Check sheet for the modelled part. Datum: model origin and axes. Units: mm. A direction names the side the tool comes from. Coordinates: 2 decimals unless noted, no trailing zeros. Loops run counter-clockwise (first coordinate to the right, second up) from the corner with the lowest first, then second, coordinate; pieces in that order, holes last. Notation, with made-up numbers: M 3,-31 L 30,-31 A22 cw 30,-19 Z; hole C -40,15.5 d8. An arc over 180 degrees is marked long. Answer in a Markdown table with one row per item. Add a question column.
```python
from build123d import *

# Parameters (mm, degrees)
BOSS_EXTRUDE2_DEPTH = 65
SKETCH4_W           = 20
SKETCH4_H           = 30
CUT_EXTRUDE1_DEPTH  = 35
SKETCH5_W           = 50
SKETCH5_H           = 80
BOSS_EXTRUDE3_DEPTH = 30
SKETCH6_W           = 30
SKETCH6_H           = 25
CUT_EXTRUDE2_DEPTH  = 20
LOFT3_START         = -65
LOFT3_DEPTH         = 65
LOFT3_START_2       = 25
LOFT3_2_DEPTH       = 76


with BuildPart() as part:
    # Sketch3 → Boss-Extrude2 (new body)
    with BuildSketch(Plane.XY):
        Polygon((0, 0), (100, 0), (100, 20), (25, 20), (25, 80), (0, 80), align=None)
    extrude(amount=-BOSS_EXTRUDE2_DEPTH)

    # Sketch4 → Cut-Extrude1 (cut)
    with BuildSketch(Plane(origin=(0, 80, 0), x_dir=(1, 0, 0), z_dir=(0, 1, 0))):
        with Locations((15, 50)):
            Rectangle(SKETCH4_W, SKETCH4_H)
    extrude(amount=-CUT_EXTRUDE1_DEPTH, mode=Mode.SUBTRACT)

    # Sketch5 → Boss-Extrude3 (add)
    with BuildSketch(Plane.ZY):
        with Locations((-40, 40)):
            Rectangle(SKETCH5_W, SKETCH5_H)
    extrude(amount=BOSS_EXTRUDE3_DEPTH)

    # Sketch6 → Cut-Extrude2 (cut)
    with BuildSketch(Plane(origin=(25, 0, 0), x_dir=(0, 0, -1), z_dir=(1, 0, 0))):
        with Locations((50, 32.5)):
            Rectangle(SKETCH6_W, SKETCH6_H)
    extrude(amount=-CUT_EXTRUDE2_DEPTH, mode=Mode.SUBTRACT)

    # Loft3: read off the stored shape, not the designer's step
    # Loft3 outline → Loft3 (add)
    with BuildSketch(Plane.XY.offset(LOFT3_START)):
        Polygon((5, 45), (5, 20), (100, 20), (50, 45), align=None)
    extrude(amount=LOFT3_DEPTH)

    # Loft3 2 outline → Loft3 2 (cut)
    with BuildSketch(Plane.YZ.offset(LOFT3_START_2)):
        Polygon((20, 0), (45, -35), (45, 0), align=None)
    extrude(amount=LOFT3_2_DEPTH, mode=Mode.SUBTRACT)


solid = part.part
```
Q1. Thickness scan on L1, parallel to Y at x = 8, z = -62; L2, parallel to X at y = 45, z = -31; L3, parallel to Z at x = 18, y = 48.5. Record the ranges inside material, lowest first.
Q2. Cross-section at D-D (y = 34.5). Record the cut outline in (x, z).
Q3. Cross-section at B-B (x = 21.5). Record the cut outline in (y, z), plus the area to 3 significant figures.
Q4. Cross-section at A-A (y = 75). Record the cut outline in (x, z), plus the area to 4 significant figures.
Q5. Go/stop test with flat-tipped pins: pin 1 (1.5 mm diameter, centred on x = 26, z = -27.5, fed in from -Y); pin 2 (7.5 mm diameter, centred on y = 23.5, z = -5.5, fed in from -X); pin 3 (15 mm diameter, centred on y = 68, z = -49.5, fed in from +X); pin 4 (10.5 mm diameter, centred on y = 43, z = -11.5, fed in from +X). Record where each tip stops, or that it passes through.
Q6. Access from +Z, -Z, +X, -X, +Y, -Y to the whole of each face (thin tool, end or side, straight path). Record for faces 1 (the face through (53.64, 29.55, -13.37)), 2 (the face through (36, 0, -33)), 3 (the face through (-15, 39, -15)), 4 (the face through (75.4, 32.3, -40.2)), 5 (the face through (15, 62, -35)).
Q7. Cross-section at C-C (z = -54). Record the cut outline in (x, y).
Answer key:
| question | item | result |
|---|---|---|
| 1 | L1 | 0 to 45 |
| 1 | L2 | -30 to 25 |
| 1 | L3 | -35 to 0 |
| 2 | outline | M -30,-65 L 71,-65 L 71,-20.3 L 25,-20.3 L 25,0 L 0,0 L 0,-15 L -30,-15 Z |
| 3 | outline | M 0,-65 L 45,-65 L 45,-35 L 80,-35 L 80,0 L 0,0 Z |
| 3 | area | 4,150 mm^2 |
| 4 | outline | M -30,-65 L 5,-65 L 5,-35 L 25,-35 L 25,0 L 0,0 L 0,-15 L -30,-15 Z |
| 4 | area | 2,525 mm^2 |
| 5 | pin 1 | y = 0 |
| 5 | pin 2 | x = 0 |
| 5 | pin 3 | x = 5 |
| 5 | pin 4 | x = 25 |
| 6 | face 1 | +Z, +X, +Y |
| 6 | face 2 | +Z, -Z, +X, -X, -Y |
| 6 | face 3 | +Z, -X, +Y, -Y |
| 6 | face 4 | +Z, -Z, +X, +Y |
| 6 | face 5 | -Z, +X, +Y |
| 7 | outline | M -30,0 L 100,0 L 100,20 L 50,45 L 5,45 L 5,80 L -30,80 Z |
